Geometry: final body of the model. Coordinates: model frame, mm. A direction names the side the tool comes from. Give positions to 0.01 mm unless a question says otherwise; leave off trailing zeros. Write each loop counter-clockwise with the first axis right and the second up, starting at its lowest first coordinate (ties: lowest second). Pieces come first, ordered by that corner, then holes. Notation, with made-up numbers: (38.25, 60) - (57.25, 60) arc R19 ccw to (57.25, 84) - close; hole circle Ø7 at (-29, 69.25). An arc over 180 degrees is marked (long way). One line per question, with ' | ' between items. Start each with the question number.
```python
from build123d import *

# Parameters (mm, degrees)
ESQUISSE1_R             = 3
BOSS_EXTRU_1_DEPTH      = 80
CONG_2_R                = 5
ESQUISSE2_W             = 40
ESQUISSE2_H             = 4
ENL_V_MAT_EXTRU_1_DEPTH = 10


with BuildPart() as part:
    # Esquisse1 → Boss.-Extru.1 (new body)
    with BuildSketch(Plane.XY):
        with BuildLine():
            ThreePointArc((0, 379), (145.037020866, 350.150342822), (267.99347007, 267.99347007))
            Line((267.99347007, 267.99347007), (260.922402258, 260.922402258))
            ThreePointArc((260.922402258, 260.922402258), (141.210186543, 340.911547497), (0, 369))
            Line((0, 369), (0, 379))
        make_face()
        with Locations((48.81679589, 370.800378154)):
            Circle(ESQUISSE1_R, mode=Mode.SUBTRACT)
    extrude(amount=BOSS_EXTRU_1_DEPTH)

    # Congé2
    cong_2_edges = [part.edges().sort_by_distance(p)[0] for p in [
        (0, 369, 40),
        (0, 379, 40),
    ]]
    fillet(cong_2_edges, radius=CONG_2_R - 0.0001)  # a hair under: the kernel refuses the full size

    # Esquisse2 → Enlèv. mat.-Extru.1 (cut)
    with BuildSketch(Plane(origin=(0, 0, 0), x_dir=(0, 0, -1), z_dir=(0.7071067811865448, -0.7071067811865503, 0))):
        with Locations((-40, 371)):
            Rectangle(ESQUISSE2_W, ESQUISSE2_H)
    extrude(amount=-ENL_V_MAT_EXTRU_1_DEPTH, mode=Mode.SUBTRACT)


solid = part.part
```
1) Line query: L1, parallel to Y at x = 207, z = 70.5; L2, parallel to X at y = 338, z = 13.5; L3, parallel to Y at x = 250, z = 74. Output: solid intervals per line, ascending.
2) First-contact query: pin 1 Ø10 at (x, z) = (110.5, 14.5) entering from +Y; pin 2 Ø6 at (x, z) = (198, 56.5) entering from +Y; pin 3 Ø1 at (y, z) = (280, 55) entering from +X. Flat tips, straight axial feed; report the tip coordinate or a pass-through.
3) Section B-B, the plane x = 37. Output: boundary loops of the cut face in (y, z), plus the area to 3 significant figures.
4) Pull-direction query (Z, two-part tool) for faces 3 (the cylindrical face through (48.17, 367.87, 39.44)), 4 (the flat face through (259, 266, 20)), 5 (the flat face through (135, 346, 0)); classes: +Z half, -Z half, draft (parallel to the pull), parting line (faces both ways), or undercut.
5) Reachability of faces 1 (the flat face through (265, 265, 39)), 2 (the flat face through (259, 266, 60)) from +Z, -Z, +X, -X, +Y, -Y: full face, straight path, thin tool, end or side. Return the list, or none.
6) Section C-C, the plane y = 303. Output: boundary loops of the cut face in (x, z).
Answer key:
1) L1: 305.47 to 317.48 | L2: 148.04 to 171.46 | L3: 271.41 to 284.85
2) pin 1: y = 364.02 | pin 2: y = 324.99 | pin 3: x = 255.97
3) outline: (367.14, 0) - (377.19, 0) - (377.19, 80) - (367.14, 80) - close | area: 804 mm^2
4) face 3: draft | face 4: undercut | face 5: -Z half
5) face 1: +Z, -Z, +X, -Y | face 2: none
6) outline: (210.6, 0) - (227.67, 0) - (227.67, 80) - (210.6, 80) - close
